Read the model definition and answer for the solid it produces. Units are mm, in the model's axes. Face numbers are marked on the shaded views. A direction names the side the tool comes from. Coordinates: 2 decimals unless noted, no trailing zeros. Loops run counter-clockwise (first coordinate to the right, second up) from the corner with the lowest first, then second, coordinate; pieces in that order, holes last. Notation, with made-up numbers: M 80,-38.75 L 126,-38.75 A21 ccw 126,-15.75 Z; hole C -21.5,87 d2. An arc over 180 degrees is marked long. Use one line per item in the form item = value. Start each with the question number.
1. The part is cut by section A-A (z = 41). Give the vertices of the cut face in (x, y), plus the area to 3 significant figures.
2. Flat-ended cylindrical pins translate along their axes: pin 1 (5.5 mm diameter, centred on x = 25, y = -25.5, fed in from -Z); pin 2 (12 mm diameter, centred on x = -8.5, y = 15.5, fed in from +Z); pin 3 (3 mm diameter, centred on y = 24.5, z = 30.5, fed in from +X). Find the tip coordinate at first contact, or state that the pin passes through.
3. Find the intervals of material crossed by probe 1 along Y at (x, z) = (23.5, 73.5); probe 2 along Z at (x, y) = (9, -15); probe 3 along Y at (x, z) = (25, 63), in increasing order. Write a range as [from, to].
4. A tool of negligible diameter and unlimited length cuts with its end or side. For the marked faces 1, 2 and 3, from which of +Z, -Z, +X, -X, +Y, -Y can it reach the whole face along a straight path? Write none if from no direction.
5. The part is cut by section D-D (z = 78.5). Give the vertices of the cut face in (x, y), plus the area to 3 significant figures.
6. The part is cut by section C-C (x = 0). Give the vertices of the cut face in (y, z), plus the area to 3 significant figures.
7. The part is cut by section B-B (y = 0). Give the vertices of the cut face in (x, z), plus the area to 3 significant figures.
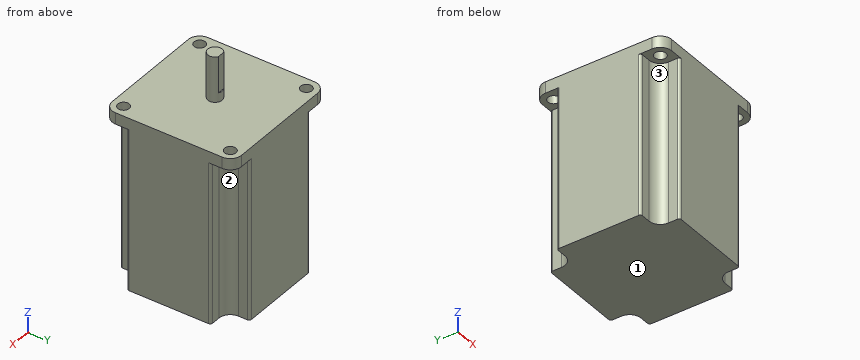
Autodesk Inventor part; units mm, degrees
ref_plane "YZ Plane" through (0, 0, 0) normal (1, 0, 0) x (0, 1, 0)
ref_plane "XZ Plane" through (0, 0, 0) normal (0, 1, 0) x (-1, 0, 0)
ref_plane "XY Plane" through (0, 0, 0) normal (0, 0, 1) x (1, 0, 0)
sketch "Sketch1" plane through (0, 0, 0) normal (0, 0, 1) x (1, 0, 0)
  line L0 (17.5, 28.5) -> (-17.5, 28.5)
  line L1 (-28.5, 17.5) -> (-28.5, -17.5)
  line L2 (28.5, -17.5) -> (28.5, 17.5)
  arc A0 (-18.5, -23.5) -> (-23.5, -18.5) centre (-23.5, -23.5) ccw
  arc A1 (23.5, -18.5) -> (18.5, -23.5) centre (23.5, -23.5) ccw
  arc A2 (18.5, 23.5) -> (23.5, 18.5) centre (23.5, 23.5) ccw
  arc A3 (-23.5, 18.5) -> (-18.5, 23.5) centre (-23.5, 23.5) ccw
  line L3 (-23.5, 18.5) -> (-27.5, 18.5)
  line L4 (-18.5, 23.5) -> (-18.5, 27.5)
  line L5 (-23.5, -18.5) -> (-27.5, -18.5)
  line L6 (-18.5, -23.5) -> (-18.5, -27.5)
  line L7 (18.5, -23.5) -> (18.5, -27.5)
  line L8 (23.5, -18.5) -> (27.5, -18.5)
  line L9 (18.5, 23.5) -> (18.5, 27.5)
  line L10 (23.5, 18.5) -> (27.5, 18.5)
  line L11 (-17.5, -28.5) -> (17.5, -28.5)
  arc A4 (-28.5, -17.5) -> (-27.5, -18.5) centre (-27.5, -17.5) ccw
  arc A5 (17.5, -28.5) -> (18.5, -27.5) centre (17.5, -27.5) ccw
  arc A6 (-27.5, 18.5) -> (-28.5, 17.5) centre (-27.5, 17.5) ccw
  arc A7 (-17.5, 28.5) -> (-18.5, 27.5) centre (-17.5, 27.5) ccw
  arc A8 (-18.5, -27.5) -> (-17.5, -28.5) centre (-17.5, -27.5) ccw
  arc A9 (28.5, 17.5) -> (27.5, 18.5) centre (27.5, 17.5) ccw
  arc A10 (18.5, 27.5) -> (17.5, 28.5) centre (17.5, 27.5) ccw
  arc A11 (27.5, -18.5) -> (28.5, -17.5) centre (27.5, -17.5) ccw
  point P0 (0, 0)
  point P1 (18.5, 28.5)
  point P2 (-18.5, -28.5)
  point P3 (28.5, -18.5)
  point P4 (28.5, 18.5)
  dimension "d2" = 28.5
  dimension "d3" = 28.5
  dimension "d4" = 10
  dimension "d5" = 10
  dimension "d6" = 10
  dimension "d7" = 10
  dimension "d8" = 57
  dimension "d9" = 57
  dimension "d10" = 1
extrude "Extrusion1" add sketch "Sketch1" along normal blind 15
sketch "Sketch2" plane through (0, 0, 15) normal (0, 0, 1) x (1, 0, 0)
  line L0 (17.5, 28.5) -> (-17.5, 28.5)
  arc A0 (-23.5, 18.5) -> (-18.5, 23.5) centre (-23.5, 23.5) ccw
  arc A1 (-23.5, 18.5) -> (-18.5, 23.5) centre (-23.5, 23.5) ccw
  line L1 (-23.5, 18.5) -> (-27.5, 18.5)
  arc A2 (-27.5, 18.5) -> (-28.5, 17.5) centre (-27.5, 17.5) ccw
  line L2 (-28.5, 17.5) -> (-28.5, -17.5)
  arc A3 (-28.5, -17.5) -> (-27.5, -18.5) centre (-27.5, -17.5) ccw
  line L3 (-27.5, -18.5) -> (-23.5, -18.5)
  arc A4 (-18.5, -23.5) -> (-23.5, -18.5) centre (-23.5, -23.5) ccw
  line L4 (-18.5, -23.5) -> (-18.5, -27.5)
  arc A5 (-18.5, -27.5) -> (-17.5, -28.5) centre (-17.5, -27.5) ccw
  line L5 (-17.5, -28.5) -> (17.5, -28.5)
  arc A6 (17.5, -28.5) -> (18.5, -27.5) centre (17.5, -27.5) ccw
  line L6 (18.5, -27.5) -> (18.5, -23.5)
  arc A7 (23.5, -18.5) -> (18.5, -23.5) centre (23.5, -23.5) ccw
  line L7 (23.5, -18.5) -> (27.5, -18.5)
  arc A8 (27.5, -18.5) -> (28.5, -17.5) centre (27.5, -17.5) ccw
  line L8 (28.5, -17.5) -> (28.5, 17.5)
  arc A9 (28.5, 17.5) -> (27.5, 18.5) centre (27.5, 17.5) ccw
  line L9 (27.5, 18.5) -> (23.5, 18.5)
  arc A10 (18.5, 23.5) -> (23.5, 18.5) centre (23.5, 23.5) ccw
  line L10 (18.5, 23.5) -> (18.5, 27.5)
  arc A11 (18.5, 27.5) -> (17.5, 28.5) centre (17.5, 27.5) ccw
  line L11 (17.5, 28.5) -> (-17.5, 28.5)
  arc A12 (-17.5, 28.5) -> (-18.5, 27.5) centre (-17.5, 27.5) ccw
  line L12 (-18.5, 27.5) -> (-18.5, 23.5)
  point P0 (0, 0)
extrude "Extrusion2" add sketch "Sketch2" along normal blind 46
sketch "Sketch3" plane through (0, 0, 61) normal (0, 0, 1) x (1, 0, 0)
  arc A0 (-23.5, 18.5) -> (-18.5, 23.5) centre (-23.5, 23.5) ccw
  line L0 (-23.5, 18.5) -> (-27.5, 18.5)
  arc A1 (-27.5, 18.5) -> (-28.5, 17.5) centre (-27.5, 17.5) ccw
  line L1 (-28.5, 17.5) -> (-28.5, -17.5)
  arc A2 (-28.5, -17.5) -> (-27.5, -18.5) centre (-27.5, -17.5) ccw
  line L2 (-27.5, -18.5) -> (-23.5, -18.5)
  arc A3 (-18.5, -23.5) -> (-23.5, -18.5) centre (-23.5, -23.5) ccw
  line L3 (-18.5, -23.5) -> (-18.5, -27.5)
  arc A4 (-18.5, -27.5) -> (-17.5, -28.5) centre (-17.5, -27.5) ccw
  line L4 (-17.5, -28.5) -> (17.5, -28.5)
  arc A5 (17.5, -28.5) -> (18.5, -27.5) centre (17.5, -27.5) ccw
  line L5 (18.5, -27.5) -> (18.5, -23.5)
  arc A6 (23.5, -18.5) -> (18.5, -23.5) centre (23.5, -23.5) ccw
  line L6 (23.5, -18.5) -> (27.5, -18.5)
  arc A7 (27.5, -18.5) -> (28.5, -17.5) centre (27.5, -17.5) ccw
  line L7 (28.5, -17.5) -> (28.5, 17.5)
  arc A8 (28.5, 17.5) -> (27.5, 18.5) centre (27.5, 17.5) ccw
  line L8 (27.5, 18.5) -> (23.5, 18.5)
  arc A9 (18.5, 23.5) -> (23.5, 18.5) centre (23.5, 23.5) ccw
  line L9 (18.5, 23.5) -> (18.5, 27.5)
  arc A10 (18.5, 27.5) -> (17.5, 28.5) centre (17.5, 27.5) ccw
  line L10 (17.5, 28.5) -> (-17.5, 28.5)
  arc A11 (-17.5, 28.5) -> (-18.5, 27.5) centre (-17.5, 27.5) ccw
  line L11 (-18.5, 27.5) -> (-18.5, 23.5)
  point P0 (0, 0)
extrude "Extrusion3" add sketch "Sketch3" along normal blind 10
sketch "Sketch4" plane through (0, 0, 71) normal (0, 0, 1) x (1, 0, 0)
  line L0 (-23.5, -28.5) -> (23.5, -28.5)
  line L1 (28.5, -23.5) -> (28.5, 23.5)
  line L2 (23.5, 28.5) -> (-23.5, 28.5)
  line L3 (-28.5, 23.5) -> (-28.5, -23.5)
  line L4 (-27.0355, -27.0355) -> (28.5, 28.5) construction
  line L5 (28.5, -28.5) -> (-28.5, 28.5) construction
  arc A0 (-23.5, 28.5) -> (-28.5, 23.5) centre (-23.5, 23.5) ccw
  arc A1 (28.5, 23.5) -> (23.5, 28.5) centre (23.5, 23.5) ccw
  arc A2 (23.5, -28.5) -> (28.5, -23.5) centre (23.5, -23.5) ccw
  arc A3 (-28.5, -23.5) -> (-23.5, -28.5) centre (-23.5, -23.5) ccw
  line L6 (17.5, 28.5) -> (-17.5, 28.5)
  circle A4 centre (-23.5, 23.5) radius 2.5
  circle A5 centre (23.5, 23.5) radius 2.5
  circle A6 centre (23.5, -23.5) radius 2.5
  circle A7 centre (-23.5, -23.5) radius 2.5
  point P0 (0, 0)
  dimension "d17" = 57
  dimension "d18" = 10
  dimension "d19" = 10
  dimension "d20" = 10
  dimension "d21" = 10
  dimension "d22" = 28.5
  dimension "d23" = 5
  dimension "d24" = 5
  dimension "d25" = 5
  dimension "d26" = 5
extrude "Extrusion4" add sketch "Sketch4" along normal blind 5
sketch "Sketch5" plane through (0, 0, 76) normal (0, 0, 1) x (1, 0, 0)
  circle A0 centre (0, 0) radius 3.15
  dimension "d29" = 6.3
extrude "Extrusion5" add sketch "Sketch5" along normal blind 20
sketch "Sketch6" plane through (0, 0, 96) normal (0, 0, 1) x (1, 0, 0)
  arc A0 (1.7029, 2.65) -> (-1.7029, 2.65) centre (0, 0) ccw
  line L0 (1.7029, 2.65) -> (-1.7029, 2.65)
  circle A1 centre (0, 0) radius 3.15
  arc A2 (1.7029, 2.65) -> (-1.7029, 2.65) centre (0, 0) ccw
extrude "Extrusion6" cut sketch "Sketch6" against normal blind 16 contours L0 A0
properties part number "Stepper motor"
Computed values:
q1.outline = M -28.5,-17.5 A1 ccw -27.5,-18.5 L -23.5,-18.5 A5 cw -18.5,-23.5 L -18.5,-27.5 A1 ccw -17.5,-28.5 L 17.5,-28.5 A1 ccw 18.5,-27.5 L 18.5,-23.5 A5 cw 23.5,-18.5 L 27.5,-18.5 A1 ccw 28.5,-17.5 L 28.5,17.5 A1 ccw 27.5,18.5 L 23.5,18.5 A5 cw 18.5,23.5 L 18.5,27.5 A1 ccw 17.5,28.5 L -17.5,28.5 A1 ccw -18.5,27.5 L -18.5,23.5 A5 cw -23.5,18.5 L -27.5,18.5 A1 ccw -28.5,17.5 Z
q1.area = 2,870 mm²
q2.pin_1 = 71
q2.pin_2 = 76
q2.pin_3 = 18.53
q3.probe_1 = [-28.5, -26], [-21, 21], [26, 28.5]
q3.probe_2 = [0, 76]
q3.probe_3 = [-18.5, 18.5]
q4.face_1 = -Z, +X, -X, +Y, -Y
q4.face_2 = -Z, +X, +Y
q4.face_3 = -Z, -X, -Y
q5.outline = C 0,0 d6.3
q5.area = 31.2 mm²
q6.outline = M -28.5,0 L 28.5,0 L 28.5,76 L 3.15,76 L 3.15,80 L 2.65,80 L 2.65,96 L -3.15,96 L -3.15,76 L -28.5,76 Z
q6.area = 4,450 mm²
q7.outline = M -28.5,0 L 28.5,0 L 28.5,76 L 3.15,76 L 3.15,96 L -3.15,96 L -3.15,76 L -28.5,76 Z
q7.area = 4,460 mm²
